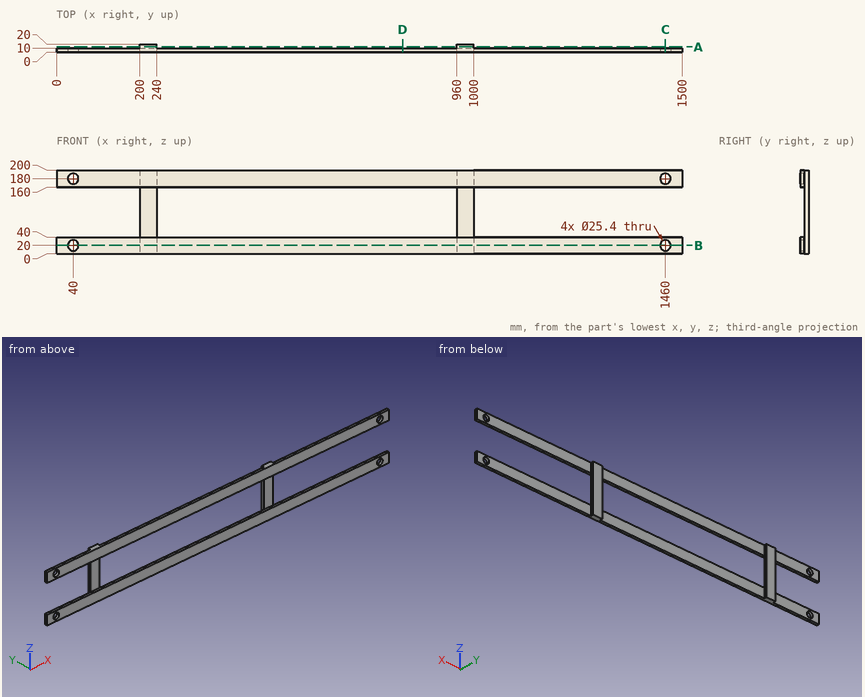
Can you work these out from the drawing? Everything is in mm from the part's minimum corner. Give positions to 0.01 mm unless a question says otherwise; leave off trailing zeros. Order: outer loops, then holes, each group sorted by start corner. A loop starts at its lowest first (then second) coordinate and runs counter-clockwise, first axis right, second up.
Item 1: I need wall thicknesses on line 1 (Z direction, x = 1460, y = 4.75); line 2 (X direction, y = 2, z = 180); line 3 (Z direction, x = 190, y = 9). Which ranges of each line are inside material? Lowest first, please.
Item 2: If we section it at D-D, the plane x = 830: Write out the boundary of the cut face in (y, z).
Item 3: If we section it at C-C, the plane x = 1460: Write out the boundary of the cut face in (y, z).
Item 4: If we section it at A-A, the plane y = 13: Write out the boundary of the cut face in (x, z).
Item 5: I'm going to push flat-ended pins straight in: pin 1 (1.5 mm diameter, centred on y = 12, z = 88, fed in from -X); pin 2 (8 mm diameter, centred on y = 15, z = 63.5, fed in from +X); pin 3 (6 mm diameter, centred on x = 152, z = 29, fed in from +Y). Where does each tip first touch, or does it pass through?
Item 6: If we section it at B-B, the plane z = 20: Write out the boundary of the cut face in (x, y).
Values:
1. line 1: z = 0 to 7.3, 32.7 to 40, 160 to 167.3, 192.7 to 200
1. line 2: x = 0 to 27.3, 52.7 to 1447.3, 1472.7 to 1500
1. line 3: z = 0 to 40, 160 to 200
2. outline: (0, 0) - (10, 0) - (10, 40) - (0, 40) - close; (0, 160) - (10, 160) - (10, 200) - (0, 200) - close
3. outline: (0, 0) - (10, 0) - (10, 7.3) - (0, 7.3) - close; (0, 32.7) - (10, 32.7) - (10, 40) - (0, 40) - close; (0, 160) - (10, 160) - (10, 167.3) - (0, 167.3) - close; (0, 192.7) - (10, 192.7) - (10, 200) - (0, 200) - close
4. outline: (200, 0) - (240, 0) - (240, 200) - (200, 200) - close; (960, 0) - (1000, 0) - (1000, 200) - (960, 200) - close
5. pin 1: stops at x = 200
5. pin 2: stops at x = 1000
5. pin 3: stops at y = 10
6. outline: (0, 0) - (27.3, 0) - (27.3, 10) - (0, 10) - close; (52.7, 0) - (1447.3, 0) - (1447.3, 10) - (1000, 10) - (1000, 20) - (960, 20) - (960, 10) - (240, 10) - (240, 20) - (200, 20) - (200, 10) - (52.7, 10) - close; (1472.7, 0) - (1500, 0) - (1500, 10) - (1472.7, 10) - close
